CAD build for the part. Positions are in the model's coordinates, mm. A direction names the side the tool comes from. Round coordinates to 2 decimals unless told otherwise and drop trailing zeros. Write each loop counter-clockwise with the first axis right and the second up, starting at its lowest first coordinate (ties: lowest second). Pieces come first, ordered by that corner, then holes. Notation, with made-up numbers: (82.25, -32.5) - (130.25, -32.5) arc R20 ccw to (130.25, -10.5) - close; hole circle Ø6 at (-12, 31.25). An arc over 180 degrees is marked (long way). Put each result on its own line as item: value. Start each with the question number.
Item 1: Mould opens along X. For faces 4 (the cylindrical face through (59.43, -3, 24.49)), 5 (the cylindrical face through (56.5, -34.5, 23.8)), 6 (the flat face through (56, 3, 49.3)) say: released by +X, released by -X, zero draft, split by the parting line, or undercut.
Item 2: Cut at B-B (y = 28.5). Give the cut face in (x, z).
Item 3: Pin check, flat tips, straight feed: pin 1 Ø14.5 at (x, z) = (87, 28.5) entering from -Y; pin 2 Ø3 at (y, z) = (25, 41.5) entering from -X; pin 3 Ø4 at (x, z) = (85.5, 34.5) entering from +Y. Stop position of each tip, or through.
Item 4: 3-axis set-ups, long thin cutter, end or side, ignore diameter. For faces 1 (the flat face through (25, 1.5, 24)), 2 (the flat face through (55, -20, 24)), 3 (the flat face through (88, 1.5, 24)): which of +Z, -Z, +X, -X, +Y, -Y reach the whole face in a straight line?
Item 5: Cut at A-A (z = 17). Give the cut face in (x, y).
Item 6: Cut at C-C (x = 70.5). Give the cut face in (y, z), and give its area (3 significant figures).
Item 7: Drill centre lines: line 1 (Y direction, x = 56.5, z = 19); line 2 (X direction, y = -27.5, z = 37); line 3 (Y direction, x = 100, z = 41.5). Where is each one in solid material? Low to high. Write a range as from..to.
```python
from build123d import *

# Parameters (mm, degrees)
F1_DEPTH = 49.3
F2_R     = 5
F4_D     = 3
F5_R     = 1
F6_R     = 4.3076910369
F7_DEPTH = 15.71207
F8_D     = 5


with BuildPart() as f1:
    # F0 (on Top) → F1 (new body)
    with BuildSketch(Plane.XY):
        with BuildLine():
            ThreePointArc((0, 1.5), (-1.5, 0), (0, -1.5))
            Line((0, -1.5), (55, -1.5))
            Line((55, -1.5), (55, -33))
            ThreePointArc((55, -33), (56.5, -34.5), (58, -33))
            Line((58, -33), (58, -1.5))
            Line((58, -1.5), (113, -1.5))
            ThreePointArc((113, -1.5), (114.5, 0), (113, 1.5))
            Line((113, 1.5), (58, 1.5))
            Line((58, 1.5), (58, 33))
            ThreePointArc((58, 33), (56.5, 34.5), (55, 33))
            Line((55, 33), (55, 1.5))
            Line((55, 1.5), (0, 1.5))
        make_face()
    extrude(amount=F1_DEPTH)

    # F2
    f2_edges = [f1.edges().sort_by_distance(p)[0] for p in [
        (58, -1.5, 24.65),
        (55, -1.5, 24.65),
        (55, 1.5, 24.65),
        (58, 1.5, 24.65),
    ]]
    fillet(f2_edges, radius=F2_R)

    # F4 (through all)
    with Locations(Plane.XY.offset(49.3)):
        with Locations((56.5, 0)):
            Hole(F4_D / 2)

    # F5
    f5_edges = [f1.edges().sort_by_distance(p)[0] for p in [
        (25, -1.5, 49.3),
        (53.535534, -2.964466, 49.3),
        (-1.5, 0, 49.3),
        (55, -19.75, 49.3),
        (25, 1.5, 49.3),
        (56.5, -34.5, 49.3),
        (53.535534, 2.964466, 49.3),
        (58, -19.75, 49.3),
        (55, 19.75, 49.3),
        (59.464466, -2.964466, 49.3),
        (56.5, 34.5, 49.3),
        (88, -1.5, 49.3),
        (58, 19.75, 49.3),
        (114.5, 0, 49.3),
        (59.464466, 2.964466, 49.3),
        (88, 1.5, 49.3),
        (55, 0, 49.3),
    ]]
    fillet(f5_edges, radius=F5_R)

    # F6 (on face) → F7 (join)
    with BuildSketch(Plane(origin=(0, 1.5, 0), x_dir=(-1, 0, 0), z_dir=(0, 1, 0))):
        with Locations((-104.8107147217, 11.4163886756)):
            Circle(F6_R)
    extrude(amount=-F7_DEPTH)

    # F8 (through all)
    with Locations(Plane.XZ.offset(1.5)):
        with Locations((22.5091800094, 10.1744234562)):
            Hole(F8_D / 2)


solid = f1.part
```
Output values:
1. face 4: undercut
1. face 5: split by the parting line
1. face 6: zero draft
2. outline: (55, 0) - (58, 0) - (58, 48.3) arc R1 ccw to (57, 49.3) - (56, 49.3) arc R1 ccw to (55, 48.3) - close
3. pin 1: y = -1.5
3. pin 2: x = 55
3. pin 3: y = 1.5
4. face 1: +Z, -Z, -X, +Y
4. face 2: +Z, -Z, -X, -Y
4. face 3: +Z, -Z, +X, +Y
5. outline: (0, -1.5) - (50, -1.5) arc R5 cw to (55, -6.5) - (55, -33) arc R1.5 ccw to (58, -33) - (58, -6.5) arc R5 cw to (63, -1.5) - (113, -1.5) arc R1.5 ccw to (113, 1.5) - (63, 1.5) arc R5 cw to (58, 6.5) - (58, 33) arc R1.5 ccw to (55, 33) - (55, 6.5) arc R5 cw to (50, 1.5) - (0, 1.5) arc R1.5 ccw to start; hole circle Ø3 at (56.5, 0)
6. outline: (-1.5, 0) - (1.5, 0) - (1.5, 48.3) arc R1 ccw to (0.5, 49.3) - (-0.5, 49.3) arc R1 ccw to (-1.5, 48.3) - close
6. area: 147 mm2
7. line 1: -34.5..-1.5, 1.5..34.5
7. line 2: 55..58
7. line 3: -1.5..1.5
